from build123d import *

# Parameters (mm, degrees)
BOSS_EXTRUDE2_DEPTH = 11.5
SKETCH5_R           = 1
BOSS_EXTRUDE5_DEPTH = 2
SKETCH3_R           = 1
BOSS_EXTRUDE6_DEPTH = 2


with BuildPart() as part:
    # Sketch1 → Boss-Extrude2 (new body)
    with BuildSketch(Plane.XY):
        with BuildLine():
            Line((0, 0), (1, 0))
            Line((1, 0), (1, 10))
            ThreePointArc((1, 10), (0.707106781, 10.707106781), (0, 11))
            Line((0, 11), (-12, 11))
            Line((-12, 11), (-12, 10))
            Line((-12, 10), (-0.5, 10))
            ThreePointArc((-0.5, 10), (-0.146446609, 9.853553391), (0, 9.5))
            Line((0, 9.5), (0, 0))
        make_face()
    extrude(amount=BOSS_EXTRUDE2_DEPTH)

    # Sketch5 → Boss-Extrude5 (add)
    with BuildSketch(Plane.ZY.offset(12)):
        with BuildLine():
            Line((7.5, 11), (10.5, 11))
            Line((10.5, 11), (10.5, 12.2))
            ThreePointArc((10.5, 12.2), (9, 13.7), (7.5, 12.2))
            Line((7.5, 12.2), (7.5, 11))
        make_face()
        with Locations(Location((9, 12.2, 0), (0, 0, 270))):
            Circle(SKETCH5_R, mode=Mode.SUBTRACT)
    boss_extrude5 = extrude(amount=-BOSS_EXTRUDE5_DEPTH)

    # Sketch3 → Boss-Extrude6 (add)
    with BuildSketch(Plane(origin=(0, 0.1, 0), x_dir=(-1, 0, 0), z_dir=(0, -1, 0))):
        with BuildLine():
            Line((-1, -10.5), (-1, -7.5))
            Line((-1, -7.5), (-2.2, -7.5))
            ThreePointArc((-2.2, -7.5), (-3.7, -9), (-2.2, -10.5))
            Line((-2.2, -10.5), (-1, -10.5))
        make_face()
        with Locations(Location((-2.2, -9, 0), (0, 0, 90))):
            Circle(SKETCH3_R, mode=Mode.SUBTRACT)
    boss_extrude6 = extrude(amount=-BOSS_EXTRUDE6_DEPTH)

    # Mirror1: Boss-Extrude5, Boss-Extrude6 across plane
    add(boss_extrude5.mirror(Plane(origin=(0, 0, 5.75), x_dir=(1, 0, 0), z_dir=(0, 0, -1))))
    add(boss_extrude6.mirror(Plane(origin=(0, 0, 5.75), x_dir=(1, 0, 0), z_dir=(0, 0, -1))))


solid = part.part
Here's how the part is built. I have some questions about the finished solid (model axes, mm). A direction names the side the tool comes from. Give positions to 0.01 mm unless a question says otherwise; leave off trailing zeros. Order: outer loops, then holes, each group sorted by start corner. A loop starts at its lowest first (then second) coordinate and runs counter-clockwise, first axis right, second up. Notation, with made-up numbers: (-3, 26.5) -> (26, 26.5) arc R26 cw to (26, 41.5) -> close; hole circle Ø9 at (31.25, 49). An arc over 180 degrees is marked (long way). One line per item, written item: value. Start each with the question number.
1. We'd pull the mould along X, two halves only. Please class faces 1 (the face through (-10, 13, 8)), 2 (the face through (2, 1, 1)), 3 (the face through (2.876, 1.086, 1.763)): released by +X, released by -X, zero draft, split by the parting line, or undercut.
2. For faces 4 (the face through (2, 1, 7.5)), 5 (the face through (3, 0.1, 8)), 6 (the face through (3, 2.1, 8)), 7 (the face through (-6, 10, 6)), which set-ups out of +Z, -Z, +X, -X, +Y, -Y let a thin tool reach every point of the face, with its end or its side?
3. Imagine slicing it at B-B, the plane x = 1.75. List the corners of the cut face in (y, z) for me, plus the area to 3 significant figures.
4. Imagine slicing it at A-A, the plane z = 2.5. List the corners of the cut face in (x, y) for me, plus the area to 3 significant figures.
5. I need wall thicknesses on probe 1 along Z at (x, y) = (-10.45, 12.2); probe 2 along X at (y, z) = (1.15, 2.5); probe 3 along Y at (x, z) = (-11.25, 2.5). Which ranges of each line are inside material? Lowest first, please. Write a range as from..to.
6. Imagine slicing it at D-D, the plane z = 10.25. List the corners of the cut face in (x, y) for me, plus the area to 3 significant figures.
7. Imagine slicing it at C-C, the plane y = 12. List the corners of the cut face in (x, z) for me, plus the area to 3 significant figures.
8. Will these pins go through, and if not, where does the flat tip stop? pin 1 Ø2 at (y, z) = (8, 6.5) entering from +X; pin 2 Ø6 at (x, z) = (-7.5, 6.5) entering from -Y; pin 3 Ø0.6 at (x, y) = (1.5, 1.5) entering from +Z.
Values follow:
1. face 1: released by +X
1. face 2: zero draft
1. face 3: undercut
2. face 4: +X, +Y, -Y
2. face 5: +Z, -Z, +X, -Y
2. face 6: +Z, -Z, +X, +Y
2. face 7: +Z, -Z, -X, -Y
3. outline: (0.1, 1) -> (2.1, 1) -> (2.1, 1.61) -> (0.1, 1.61) -> close; (0.1, 3.39) -> (2.1, 3.39) -> (2.1, 4) -> (0.1, 4) -> close; (0.1, 7.5) -> (2.1, 7.5) -> (2.1, 8.11) -> (0.1, 8.11) -> close; (0.1, 9.89) -> (2.1, 9.89) -> (2.1, 10.5) -> (0.1, 10.5) -> close
3. area: 4.86 mm2
4. outline: (-12, 10) -> (-0.5, 10) arc R0.5 cw to (0, 9.5) -> (0, 0) -> (1, 0) -> (1, 0.1) -> (1.2, 0.1) -> (1.2, 2.1) -> (1, 2.1) -> (1, 10) arc R1 ccw to (0, 11) -> (-10, 11) -> (-10, 11.2) -> (-12, 11.2) -> close; (-12, 13.2) -> (-10, 13.2) -> (-10, 13.7) -> (-12, 13.7) -> close; (3.2, 0.1) -> (3.7, 0.1) -> (3.7, 2.1) -> (3.2, 2.1) -> close
4. area: 25.6 mm2
5. probe 1: z = 1..1.5, 3.5..4, 7.5..8, 10..10.5
5. probe 2: x = 0..1.2, 3.2..3.7
5. probe 3: y = 10..11.2, 13.2..13.7
6. outline: (-12, 10) -> (-0.5, 10) arc R0.5 cw to (0, 9.5) -> (0, 0) -> (1, 0) -> (1, 0.1) -> (3.03, 0.1) -> (3.03, 2.1) -> (1, 2.1) -> (1, 10) arc R1 ccw to (0, 11) -> (-10, 11) -> (-10, 13.03) -> (-12, 13.03) -> close
6. area: 31.0 mm2
7. outline: (-12, 1) -> (-10, 1) -> (-10, 1.52) -> (-12, 1.52) -> close; (-12, 3.48) -> (-10, 3.48) -> (-10, 4) -> (-12, 4) -> close; (-12, 7.5) -> (-10, 7.5) -> (-10, 8.02) -> (-12, 8.02) -> close; (-12, 9.98) -> (-10, 9.98) -> (-10, 10.5) -> (-12, 10.5) -> close
7. area: 4.16 mm2
8. pin 1: stops at x = 1
8. pin 2: stops at y = 10
8. pin 3: stops at z = 10.5
